from build123d import *

# Parameters (mm, degrees)
BOX021_W     = 10
BOX021_H     = 10
BOX021_DEPTH = 31
BOX020_W     = 10
BOX020_H     = 10
BOX020_DEPTH = 30
BOX019_W     = 10
BOX019_H     = 10
BOX019_DEPTH = 25
BOX018_W     = 10
BOX018_H     = 10
BOX018_DEPTH = 25
BOX010_W     = 2
BOX010_H     = 80
BOX010_DEPTH = 18
BOX011_W     = 4
BOX011_H     = 76
BOX011_DEPTH = 18


with BuildPart() as obj1:
    # Box021 → Box021 (new body)
    with BuildSketch(Plane(origin=(110, 80.8, 0), x_dir=(1, 0, 0), z_dir=(0, 0, 1))):
        with Locations((5, 5)):
            Rectangle(BOX021_W, BOX021_H)
    extrude(amount=BOX021_DEPTH)


with BuildPart() as obj2:
    # Box020 → Box020 (new body)
    with BuildSketch(Plane(origin=(109, -8.8, 0), x_dir=(1, 0, 0), z_dir=(0, 0, 1))):
        with Locations((5, 5)):
            Rectangle(BOX020_W, BOX020_H)
    extrude(amount=BOX020_DEPTH)


with BuildPart() as obj3:
    # Box019 → Box019 (new body)
    with BuildSketch(Plane(origin=(114.8, 78.8, 0), x_dir=(1, 0, 0), z_dir=(0, 0, 1))):
        with Locations((5, 5)):
            Rectangle(BOX019_W, BOX019_H)
    extrude(amount=BOX019_DEPTH)


with BuildPart() as obj4:
    # Box018 → Box018 (new body)
    with BuildSketch(Plane(origin=(114.8, -6.8, 0), x_dir=(1, 0, 0), z_dir=(0, 0, 1))):
        with Locations((5, 5)):
            Rectangle(BOX018_W, BOX018_H)
    extrude(amount=BOX018_DEPTH)


with BuildPart() as obj5:
    # Box010 → Box010 (new body)
    with BuildSketch(Plane(origin=(113, 1, 23), x_dir=(1, 0, 0), z_dir=(0, 0, 1))):
        with Locations((1, 40)):
            Rectangle(BOX010_W, BOX010_H)
    extrude(amount=BOX010_DEPTH)


with BuildPart() as front:
    # Box011 → Box011 (new body)
    with BuildSketch(Plane(origin=(113, 3, 23), x_dir=(1, 0, 0), z_dir=(0, 0, 1))):
        with Locations((2, 38)):
            Rectangle(BOX011_W, BOX011_H)
    extrude(amount=BOX011_DEPTH)

    # Fusion010: union obj5
    add(obj5.part)


with BuildPart() as front_1:
    # Fusion010 placement: moved
    add(front.part.moved(Location((0, 0, -19))))

    # Cut013: cut obj4
    add(obj4.part, mode=Mode.SUBTRACT)

    # Cut014: cut obj3
    add(obj3.part, mode=Mode.SUBTRACT)

    # Cut015: cut obj2
    add(obj2.part, mode=Mode.SUBTRACT)

    # Cut016: cut obj1
    add(obj1.part, mode=Mode.SUBTRACT)


solid = front_1.part
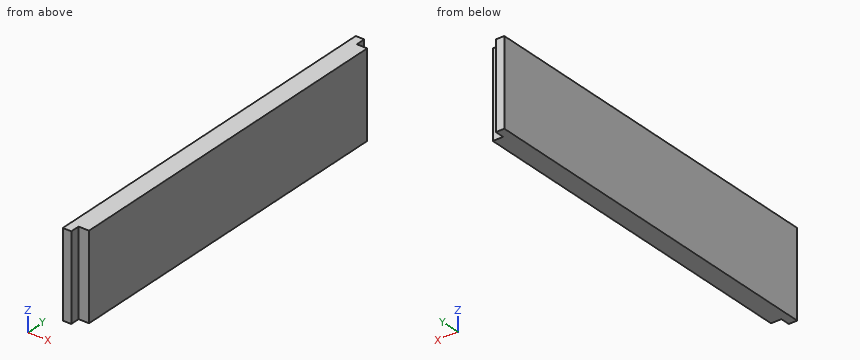
Verification items for the finished model (mm, model axes). Give positions to 0.01 mm unless a question says otherwise; leave off trailing zeros. Write each loop counter-clockwise with the first axis right and the second up, starting at its lowest first coordinate (ties: lowest second). Pieces come first, ordered by that corner, then holes.
(1) Gauge pin test, flat ends, axial feed: pin 1 (2 mm diameter, centred on y = 80, z = 17.5, fed in from +X); pin 2 (0.7 mm diameter, centred on x = 116, z = 11.5, fed in from -Y); pin 3 (1.1 mm diameter, centred on x = 116, z = 13, fed in from +Y). Record the tip position at first contact, or that the pin passes through.
(2) Material ranges on line 1 (Y direction, x = 115.9, z = 20.75), recorded low to high.
(3) Cross-section at A-A (z = 11.75). Enter the section's corners in (x, y), plus the area to 3 significant figures.
(4) Cross-section at B-B (x = 115.65). Enter the section's corners in (y, z).
Worked out:
1. pin 1: stops at x = 114.8
1. pin 2: stops at y = 3.2
1. pin 3: stops at y = 78.8
2. line 1: y = 3.2 to 78.8
3. outline: (113, 1.2) - (114.8, 1.2) - (114.8, 3.2) - (117, 3.2) - (117, 78.8) - (114.8, 78.8) - (114.8, 80.8) - (113, 80.8) - close
3. area: 310 mm2
4. outline: (3.2, 4) - (78.8, 4) - (78.8, 22) - (3.2, 22) - close
